from build123d import *

# Parameters (mm, degrees)
SKETCH_2_R          = 2.75
EXTRUDE_1_DEPTH     = 6
SKETCH_3_R          = 5
CUT_EXTRUDE_1_DEPTH = 3
FILLET_1_R          = 5
SKETCH_4_R          = 6.5
CUT_EXTRUDE_2_DEPTH = 4


with BuildPart() as part:
    # Эскиз2 → Бобышка-Вытянуть1 (new body)
    with BuildSketch(Plane.XY):
        with BuildLine():
            Line((10, 19), (10, -19))
            Line((10, -19), (-10, -19))
            Line((-10, -19), (-10, 19))
            ThreePointArc((-10, 19), (0, 29), (10, 19))
        make_face()
        with Locations((0, 1.5)):
            Circle(SKETCH_2_R, mode=Mode.SUBTRACT)
        with Locations((0, -12.5)):
            Circle(SKETCH_2_R, mode=Mode.SUBTRACT)
        with Locations((0, 19)):
            Circle(SKETCH_2_R, mode=Mode.SUBTRACT)
    extrude(amount=EXTRUDE_1_DEPTH)

    # Эскиз3 → Вырез-Вытянуть1 (cut)
    with BuildSketch(Plane.XY.offset(6)):
        with Locations((0, 1.5)):
            Circle(SKETCH_3_R)
        with Locations((0, -12.5)):
            Circle(SKETCH_3_R)
    extrude(amount=-CUT_EXTRUDE_1_DEPTH, mode=Mode.SUBTRACT)

    # Скругление1
    fillet_1_edges = [part.edges().sort_by_distance(p)[0] for p in [
        (10, -19, 3),
        (-10, -19, 3),
    ]]
    fillet(fillet_1_edges, radius=FILLET_1_R)

    # Эскиз4 → Вырез-Вытянуть2 (cut)
    with BuildSketch(Plane.XY.offset(6)):
        with Locations((0, 19)):
            Circle(SKETCH_4_R)
    extrude(amount=-CUT_EXTRUDE_2_DEPTH, mode=Mode.SUBTRACT)


solid = part.part
Work out the finished part from the listing and answer in its coordinate system (mm). A direction names the side the tool comes from. Coordinates: 2 decimals unless noted, no trailing zeros. Loops run counter-clockwise (first coordinate to the right, second up) from the corner with the lowest first, then second, coordinate; pieces in that order, holes last. Notation, with made-up numbers: (67, -27) -> (104, -27) arc R19 ccw to (104, 10) -> close; hole circle Ø3 at (24, -35.5). An arc over 180 degrees is marked (long way). Write each question's results on one line, items separated by ' | '. Start each with the question number.
1) The mould has two halves that part along X. Classify faces 3 (the flat face through (-4, 5, 6)), 4 (the cylindrical face through (0, 29, 3)), 5 (the cylindrical face through (-0.846, 25.445, 4.028)), 6 (the cylindrical face through (-8, -18, 3)): pulls with the +X half, pulls with the -X half, needs draft (parallel to the pull), parting line crosses it, or undercut.
2) Find section B-B on z = 4.45. Determine the outline of the cut face in (x, y), then the cut area to 3 significant figures.
3) Find section A-A on x = 0. Determine the outline of the cut face in (y, z).
4) Find section C-C on y = -0.5. Determine the outline of the cut face in (x, z).
5) Consider line 1 along Y through (x, z) = (0, 4.6); line 2 along Y through (x, z) = (0, 1.2); line 3 along X through (y, z) = (1.5, 1). Determine where each line is inside the solid, lowest interval first.
6) Flat-ended cylindrical pins translate along their axes: P1, Ø4.5, axis at x = 0, y = 1.5, coming from the -Z side; P2, Ø6.5, axis at x = 0, y = 19, coming from the +Z side; P3, Ø3, axis at x = -1, y = -11, coming from the +Z side; P4, Ø6, axis at x = 0, y = -12.5, coming from the -Z side. Find the tip coordinate at first contact, or state that the pin passes through.
7) For faces 1 (the flat face through (0, 5, 0)), 2 (the cylindrical face through (2.688, 5.716, 4.521)), determine the directions among +Z, -Z, +X, -X, +Y, -Y from which every point of the face is accessible in a straight line to the end or side of a thin tool.
8) Find section D-D on y = 13. Determine the outline of the cut face in (x, z), then the cut area to 3 significant figures.
Response values:
1) face 3: needs draft | face 4: parting line crosses it | face 5: undercut | face 6: pulls with the -X half
2) outline: (-10, -14) arc R5 ccw to (-5, -19) -> (5, -19) arc R5 ccw to (10, -14) -> (10, 19) arc R10 ccw to (-10, 19) -> close; hole circle Ø13 at (0, 19); hole circle Ø10 at (0, -12.5); hole circle Ø10 at (0, 1.5) | area: 617 mm^2
3) outline: (-19, 0) -> (-15.25, 0) -> (-15.25, 3) -> (-17.5, 3) -> (-17.5, 6) -> (-19, 6) -> close; (-9.75, 0) -> (-1.25, 0) -> (-1.25, 3) -> (-3.5, 3) -> (-3.5, 6) -> (-7.5, 6) -> (-7.5, 3) -> (-9.75, 3) -> close; (4.25, 0) -> (16.25, 0) -> (16.25, 2) -> (12.5, 2) -> (12.5, 6) -> (6.5, 6) -> (6.5, 3) -> (4.25, 3) -> close; (21.75, 0) -> (29, 0) -> (29, 6) -> (25.5, 6) -> (25.5, 2) -> (21.75, 2) -> close
4) outline: (-10, 0) -> (-1.89, 0) -> (-1.89, 3) -> (-4.58, 3) -> (-4.58, 6) -> (-10, 6) -> close; (1.89, 0) -> (10, 0) -> (10, 6) -> (4.58, 6) -> (4.58, 3) -> (1.89, 3) -> close
5) line 1: y = -19 to -17.5, -7.5 to -3.5, 6.5 to 12.5, 25.5 to 29 | line 2: y = -19 to -15.25, -9.75 to -1.25, 4.25 to 16.25, 21.75 to 29 | line 3: x = -10 to -2.75, 2.75 to 10
6) P1: passes through | P2: stops at z = 2 | P3: stops at z = 3 | P4: stops at z = 0
7) face 1: -Z, +X, -X, +Y, -Y | face 2: +Z
8) outline: (-10, 0) -> (10, 0) -> (10, 6) -> (2.5, 6) -> (2.5, 2) -> (-2.5, 2) -> (-2.5, 6) -> (-10, 6) -> close | area: 100 mm^2
